from build123d import *

# Parameters (mm, degrees)
SKETCH1_R           = 120
SKETCH1_R_2         = 15
BOSS_EXTRUDE1_DEPTH = 16


with BuildPart() as part:
    # Sketch1 → Boss-Extrude1 (new body)
    with BuildSketch(Plane.XY):
        with Locations((-157.313413121, 131.73738084)):
            Circle(SKETCH1_R)
        with Locations((-157.313413121, 131.73738084)):
            Circle(SKETCH1_R_2, mode=Mode.SUBTRACT)
        with BuildLine():
            Line((-167.313413121, 103.453109593), (-167.313413121, 43.987736967))
            ThreePointArc((-167.313413121, 43.987736967), (-171.077317476, 36.170377367), (-179.535635343, 34.237776536))
            ThreePointArc((-179.535635343, 34.237776536), (-228.024091239, 61.026702722), (-254.813017425, 109.515158618))
            ThreePointArc((-254.813017425, 109.515158618), (-252.880416594, 117.973476485), (-245.063056995, 121.73738084))
            Line((-245.063056995, 121.73738084), (-185.597684368, 121.73738084))
            ThreePointArc((-185.597684368, 121.73738084), (-178.526616556, 110.524177405), (-167.313413121, 103.453109593))
        make_face(mode=Mode.SUBTRACT)
        with BuildLine():
            Line((-245.063056995, 141.73738084), (-185.597684368, 141.73738084))
            ThreePointArc((-185.597684368, 141.73738084), (-178.526616556, 152.950584276), (-167.313413121, 160.021652088))
            Line((-167.313413121, 160.021652088), (-167.313413121, 219.487024714))
            ThreePointArc((-167.313413121, 219.487024714), (-171.077317476, 227.304384314), (-179.535635343, 229.236985145))
            ThreePointArc((-179.535635343, 229.236985145), (-228.024091239, 202.448058959), (-254.813017425, 153.959603063))
            ThreePointArc((-254.813017425, 153.959603063), (-252.880416594, 145.501285196), (-245.063056995, 141.73738084))
        make_face(mode=Mode.SUBTRACT)
        with BuildLine():
            Line((-147.313413121, 219.487024714), (-147.313413121, 160.021652088))
            ThreePointArc((-147.313413121, 160.021652088), (-136.100209685, 152.950584276), (-129.029141873, 141.73738084))
            Line((-129.029141873, 141.73738084), (-69.563769247, 141.73738084))
            ThreePointArc((-69.563769247, 141.73738084), (-61.746409647, 145.501285196), (-59.813808816, 153.959603063))
            ThreePointArc((-59.813808816, 153.959603063), (-86.602735002, 202.448058959), (-135.091190899, 229.236985145))
            ThreePointArc((-135.091190899, 229.236985145), (-143.549508765, 227.304384314), (-147.313413121, 219.487024714))
        make_face(mode=Mode.SUBTRACT)
        with BuildLine():
            Line((-147.313413121, 103.453109593), (-147.313413121, 43.987736967))
            ThreePointArc((-147.313413121, 43.987736967), (-143.549508765, 36.170377367), (-135.091190899, 34.237776536))
            ThreePointArc((-135.091190899, 34.237776536), (-86.602735002, 61.026702722), (-59.813808816, 109.515158618))
            ThreePointArc((-59.813808816, 109.515158618), (-61.746409647, 117.973476485), (-69.563769247, 121.73738084))
            Line((-69.563769247, 121.73738084), (-129.029141873, 121.73738084))
            ThreePointArc((-129.029141873, 121.73738084), (-136.100209685, 110.524177405), (-147.313413121, 103.453109593))
        make_face(mode=Mode.SUBTRACT)
    extrude(amount=BOSS_EXTRUDE1_DEPTH)


solid = part.part
Source: CAD feature listing. Evaluate the final solid. Frame: model axes, mm. Give positions to 0.01 mm unless a question says otherwise; leave off trailing zeros. Order: outer loops, then holes, each group sorted by start corner. A loop starts at its lowest first (then second) coordinate and runs counter-clockwise, first axis right, second up. Notation, with made-up numbers: (77.5, -40) -> (83.5, -40) arc R22 ccw to (83.5, -4) -> close; hole circle Ø9 at (43, 83). An arc over 180 degrees is marked (long way). Use a Markdown table: item, result.
1) Section query D-D, the plane y = 236.5. Return the cut outline in (x, z), then the cut area to 3 significant figures.
Answer list:
| item | result |
|---|---|
| outline | (-215.84, 0) -> (-98.79, 0) -> (-98.79, 16) -> (-215.84, 16) -> close |
| area | 1,870 mm² |
2) Section query A-A, the plane x = -217. Return the cut outline in (y, z).
Answer list:
| item | result |
|---|---|
| outline | (27.63, 0) -> (51.5, 0) -> (51.5, 16) -> (27.63, 16) -> close; (121.74, 0) -> (141.74, 0) -> (141.74, 16) -> (121.74, 16) -> close; (211.97, 0) -> (235.84, 0) -> (235.84, 16) -> (211.97, 16) -> close |
3) Contact query for flat-ended pins moving along their axis: P1, Ø5, axis at x = -193.5, y = 224, coming from the -Z side; P2, Ø5, axis at y = 85, z = 10.5, coming from the +X side (3 decimals); P3, Ø5, axis at y = 181, z = 11.5, coming from the +X side; P4, Ø6, axis at y = 150, z = 10.5, coming from the -X side. Output: stop coordinate, or through.
Answer list:
| item | result |
|---|---|
| P1 | z = 0 |
| P2 | x = -45.765 |
| P3 | x = -46.8 |
| P4 | x = -276.34 |
4) Mould query, pull axis X, two halves, no side actions, for faces 1 (the cylindrical face through (-172.935, 250.716, 7.888)), 2 (the flat face through (-159, 107, 0)), 3 (the cylindrical face through (-170.98, 36.25, 7.89)), 4 (the cylindrical face through (-178.7, 110.7, 7.9)). Classes: +X half, -X half, draft (parallel to the pull), parting line (faces both ways), or undercut.
Answer list:
| item | result |
|---|---|
| face 1 | parting line |
| face 2 | draft |
| face 3 | undercut |
| face 4 | undercut |
5) Ray query, line 1 along Y through (x, z) = (-77, 8.25); line 2 along Y through (x, z) = (-214, 3.5); line 3 along X through (y, z) = (89.5, 14.75). Return the intervals inside material, ascending. Write a range as [from, to].
Answer list:
| item | result |
|---|---|
| line 1 | [42.58, 72.16], [121.74, 141.74], [191.32, 220.9] |
| line 2 | [25.97, 49.36], [121.74, 141.74], [214.12, 237.5] |
| line 3 | [-269.63, -247.96], [-167.31, -147.31], [-66.67, -44.99] |
6) Section query C-C, the plane y = 67. Return the cut outline in (x, z), then the cut area to 3 significant figures.
Answer list:
| item | result |
|---|---|
| outline | (-258.35, 0) -> (-233.53, 0) -> (-233.53, 16) -> (-258.35, 16) -> close; (-167.31, 0) -> (-147.31, 0) -> (-147.31, 16) -> (-167.31, 16) -> close; (-81.1, 0) -> (-56.27, 0) -> (-56.27, 16) -> (-81.1, 16) -> close |
| area | 1,110 mm² |
7) Section query B-B, the plane z = 8.5. Return the cut outline in (x, y), then the cut area to 3 significant figures.
Answer list:
| item | result |
|---|---|
| outline | circle Ø240 at (-157.31, 131.74); hole (-254.81, 109.52) arc R100 ccw to (-179.54, 34.24) arc R10 ccw to (-167.31, 43.99) -> (-167.31, 103.45) arc R30 cw to (-185.6, 121.74) -> (-245.06, 121.74) arc R10 ccw to start; hole (-254.81, 153.96) arc R10 ccw to (-245.06, 141.74) -> (-185.6, 141.74) arc R30 cw to (-167.31, 160.02) -> (-167.31, 219.49) arc R10 ccw to (-179.54, 229.24) arc R100 ccw to start; hole circle Ø30 at (-157.31, 131.74); hole (-147.31, 43.99) arc R10 ccw to (-135.09, 34.24) arc R100 ccw to (-59.81, 109.52) arc R10 ccw to (-69.56, 121.74) -> (-129.03, 121.74) arc R30 cw to (-147.31, 103.45) -> close; hole (-147.31, 160.02) arc R30 cw to (-129.03, 141.74) -> (-69.56, 141.74) arc R10 ccw to (-59.81, 153.96) arc R100 ccw to (-135.09, 229.24) arc R10 ccw to (-147.31, 219.49) -> close |
| area | 21,800 mm² |
